Part print with two shaded views. Sizes in mm from the minimum x, y, z corner. Round coordinates to 2 decimals unless told otherwise and drop trailing zeros. Order: outer loops, then holes, each group sorted by start corner. A loop starts at its lowest first (then second) coordinate and runs counter-clockwise, first axis right, second up. Notation, with made-up numbers: (60.5, 4.25) - (82.5, 4.25) arc R18 cw to (82.5, 38.25) - close; hole circle Ø3 at (-12.75, 39). An arc over 180 degrees is marked (long way). Use one line per item in the form item = value.
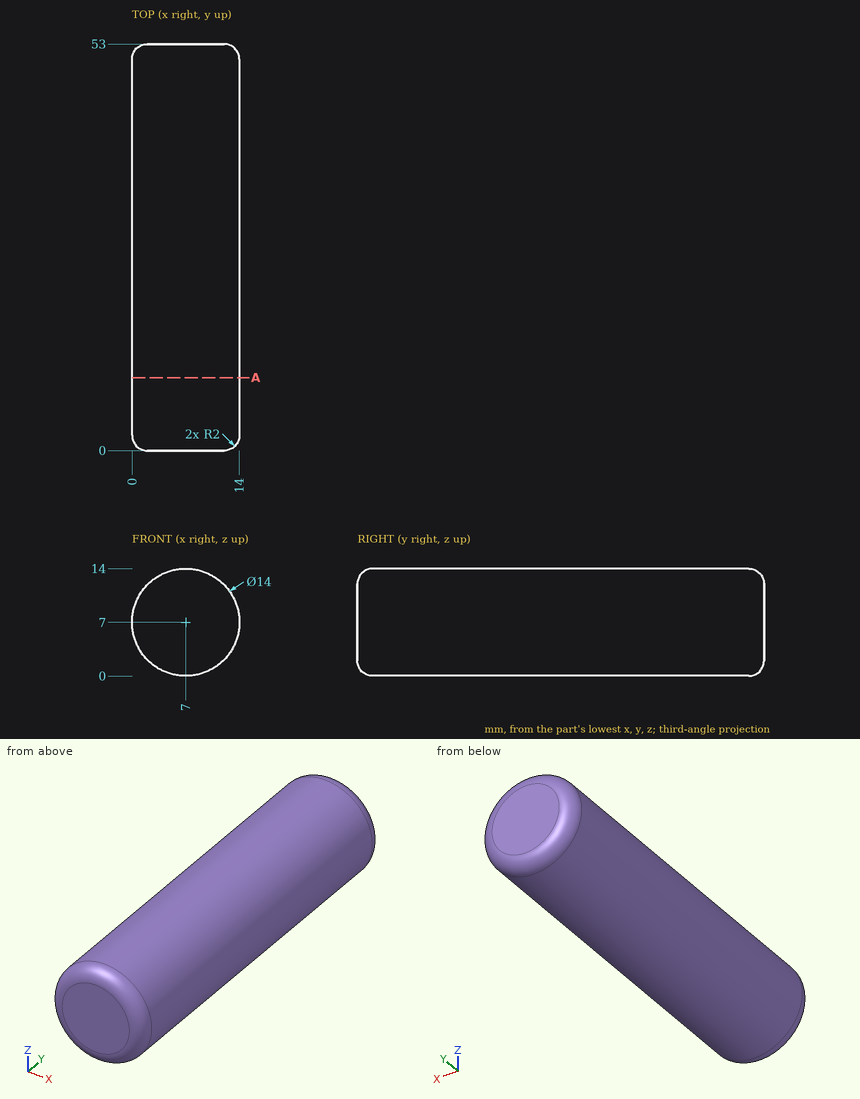
(1) Pin check, flat tips, straight feed: pin 1 (5 mm diameter, centred on y = 15.5, z = 12.5, fed in from -X); pin 2 (2 mm diameter, centred on y = 33.5, z = 3.5, fed in from +X); pin 3 (2 mm diameter, centred on x = 3.5, y = 23.5, fed in from +Z). Stop position of each tip, or through.
Report:
pin_1 = 0.68
pin_2 = 13.54
pin_3 = 13.54
(2) Slice it at A-A on y = 9.5. Give the cut face in (x, z).
Report:
outline = circle Ø14 at (7, 7)
(3) Probe probe 1 along X at (y, z) = (14.5, 7.25); probe 2 along Y at (x, z) = (9, 11.75); probe 3 along Z at (x, y) = (4.25, 47). List the from-to ranges inside material, lowest first. Write a range as [from, to].
Report:
probe_1 = [0, 14]
probe_2 = [0.01, 52.99]
probe_3 = [0.56, 13.44]
